```python
from build123d import *

# Parameters (mm, degrees)
REVOLVE1_ANGLE     = 270
CUT_EXTRUDE1_DEPTH = 151.069983674
SKETCH3_R          = 3.75
CUT_EXTRUDE2_DEPTH = 133.664991614
SKETCH5_R          = 30
CUT_EXTRUDE3_DEPTH = 151.069983674
CUT_EXTRUDE4_DEPTH = 151.06998382


with BuildPart() as part:
    # Sketch1 → Revolve1 (revolve)
    with BuildSketch(Plane.XY):
        with BuildLine():
            Line((47.5, 40), (50, 37.5))
            Line((50, 37.5), (89, 37.5))
            Line((89, 37.5), (91.5, 40))
            Line((91.5, 40), (120, 40))
            Line((120, 40), (120, 27))
            ThreePointArc((120, 27), (120.585786438, 25.585786438), (122, 25))
            Line((122, 25), (139, 25))
            Line((139, 25), (139, 0))
            Line((139, 0), (0, 0))
            Line((0, 0), (0, 25))
            Line((0, 25), (17, 25))
            ThreePointArc((17, 25), (18.414213562, 25.585786438), (19, 27))
            Line((19, 27), (19, 40))
            Line((19, 40), (47.5, 40))
        make_face()
    revolve(axis=Axis((0, 0, 0), (1, 0, 0)), revolution_arc=REVOLVE1_ANGLE)

    # Sketch2 → Cut-Extrude1 (cut, through all)
    with BuildSketch(Plane.ZY):
        with BuildLine():
            Line((0, 10), (12, 10))
            ThreePointArc((12, 10), (15, 7), (12, 4))
            Line((12, 4), (0, 4))
            ThreePointArc((0, 4), (-3, 7), (0, 10))
        make_face()
    extrude(amount=-CUT_EXTRUDE1_DEPTH, mode=Mode.SUBTRACT)

    # Sketch3 → Cut-Extrude2 (cut, through all)
    with BuildSketch(Plane(origin=(120, 0, 0), x_dir=(0, 0, -1), z_dir=(1, 0, 0))):
        with Locations((-8.282209443, 30.909626441)):
            Circle(SKETCH3_R)
        with Locations((30.909626441, -8.282209443)):
            Circle(SKETCH3_R)
        with Locations((22.627416998, -22.627416998)):
            Circle(SKETCH3_R)
        with Locations((8.282209443, -30.909626441)):
            Circle(SKETCH3_R)
        with Locations((-8.282209443, -30.909626441)):
            Circle(SKETCH3_R)
        with Locations((-22.627416998, -22.627416998)):
            Circle(SKETCH3_R)
        with Locations((-30.909626441, -8.282209443)):
            Circle(SKETCH3_R)
        with Locations((-30.909626441, 8.282209443)):
            Circle(SKETCH3_R)
        with Locations((-22.627416998, 22.627416998)):
            Circle(SKETCH3_R)
    extrude(amount=-CUT_EXTRUDE2_DEPTH, mode=Mode.SUBTRACT)

    # Sketch5 → Cut-Extrude3 (cut, through all)
    with BuildSketch(Plane(origin=(0, 0, 0), x_dir=(1, 0, 0), z_dir=(0, 1, 0))):
        with Locations((139, 40)):
            Circle(SKETCH5_R)
    extrude(amount=-CUT_EXTRUDE3_DEPTH, mode=Mode.SUBTRACT)

    # Sketch6 → Cut-Extrude4 (cut, through all)
    with BuildSketch(Plane(origin=(0, 0, 0), x_dir=(1, 0, 0), z_dir=(0, 1, 0))):
        with BuildLine():
            Line((104.531728645, 33.922313782), (109.45576741, 34.79055467))
            ThreePointArc((109.45576741, 34.79055467), (115.199399791, 21.73715713), (126.321452148, 12.810766389))
            Line((126.321452148, 12.810766389), (124.208360839, 8.279227454))
            ThreePointArc((124.208360839, 8.279227454), (111.23263309, 18.693349985), (104.531728645, 33.922313782))
        make_face()
    extrude(amount=-CUT_EXTRUDE4_DEPTH, mode=Mode.SUBTRACT)


solid = part.part
```
Could you check a few things on this model? Use its own coordinates, in mm. A direction names the side the tool comes from. Coordinates: 2 decimals unless noted, no trailing zeros. Order: outer loops, then holes, each group sorted by start corner. A loop starts at its lowest first (then second) coordinate and runs counter-clockwise, first axis right, second up. Notation, with made-up numbers: M -16,33 L 29,33 A24 cw 29,48 Z; hole C -11.75,6.5 d8. An arc over 180 degrees is marked long. Use a Markdown table: item, result. Add a question column.
Q1. I want a section at B-B on z = 31.5. Give the number of separate pieces and of enclosed holes in the cut face, then the cut area to 3 significant figures.
Q2. We'd pull the mould along X, two halves only. Please class faces 1 (the flat face through (70, 25, 0)), 2 (the flat face through (125.28, -11.63, -10.58)), 3 (the flat face through (0, -5, 6)): pulls with the +X half, pulls with the -X half, needs draft (parallel to the pull), parting line crosses it, or undercut.
Q3. I'm going to push flat-ended pins straight in: pin 1 (13 mm diameter, centred on x = 46.5, z = 7, fed in from +Y); pin 2 (4 mm diameter, centred on x = 27, y = 24, fed in from -Z); pin 3 (2 mm diameter, centred on y = -25.5, z = -9.5, fed in from +X). Where does each tip first touch, or does it pass through?
Q4. If I drill on L1, parallel to Y at x = 61.5, z = 1; L2, parallel to Z at x = 92.5, y = -30.5; L3, parallel to Y at x = 96, z = 10.5, over which ranges is the centre line in solid material (lowest first)?
Q5. Which directions (+Z, -Z, +X, -X, +Y, -Y) give clear straight access to the entire face, cutting with the end or side of a thin tool? Please do faces 4 (the conical face through (49.879, -25.711, 27.465)), 5 (the cylindrical face through (8.619, -17.085, 18.251)), 6 (the flat face through (70, 2, 0)), 7 (the cylindrical face through (111, -15, -19)).
Q6. I want a section at A-A on x = 13. List the corners of the cut face in (y, z) for me.
Checked values:
| question | item | result |
|---|---|---|
| 1 | separate pieces | 3 |
| 1 | enclosed holes | 0 |
| 1 | area | 3,130 mm² |
| 2 | face 1 | needs draft |
| 2 | face 2 | undercut |
| 2 | face 3 | pulls with the -X half |
| 3 | pin 1 | y = 40 |
| 3 | pin 2 | z = 0 |
| 3 | pin 3 | x = 120.16 |
| 4 | L1 | -37.49 to 4, 10 to 37.49 |
| 4 | L2 | -25.88 to -12.01, -4.55 to 4.55, 12.01 to 25.88 |
| 4 | L3 | -38.6 to -33.93, -27.89 to 4, 10 to 27.89, 33.93 to 38.6 |
| 5 | face 4 | none |
| 5 | face 5 | -X |
| 5 | face 6 | -Z, +X, -X, +Y |
| 5 | face 7 | +Y, -Y |
| 6 | outline | M 0,-25 L 0,0 L 4,0 L 4,12 A3 cw 10,12 L 10,0 L 25,0 A25 ccw long Z |
